Input: part model. Units: mm. Frame: model coordinates. A direction names the side the tool comes from. Round coordinates to 2 decimals unless told otherwise and drop trailing zeros. Order: outer loops, then holes, each group sorted by start corner. A loop starts at its lowest first (then second) coordinate and runs counter-clockwise, first axis right, second up. Notation, with made-up numbers: (54.5, 10.5) -> (64.5, 10.5) arc R21 cw to (64.5, 19.5) -> close; hole circle Ø2 at (-32.75, 42). An arc over 180 degrees is marked (long way). Answer as CSV lines item,"result". Start each with the question number.
1) Mould query, pull axis X, two halves, no side actions, for faces 4 (the face through (0, 5, 35)), 5 (the face through (5, 5, 65)), 6 (the face through (5, 0, 35)). Classes: +X half, -X half, draft (parallel to the pull), parting line (faces both ways), or undercut.
2) Section query D-D, the plane x = 5. Output: boundary loops of the cut face in (y, z), and give its area (3 significant figures).
3) Access query for faces 1 (the face through (6.6, 6.2, 68)), 2 (the face through (7, 5, 3)), 3 (the face through (7.2, 5.1, 0)). Directions: +Z, -Z, +X, -X, +Y, -Y. A direction counts if a zero-diameter tool reaches every point of the face in a straight line with its end or side. Return the directions, or none.
4) First-contact query: P1, Ø1.2, axis at x = 5.5, y = 5.5, coming from the -Z side; P2, Ø1, axis at x = 6, z = 54.5, coming from the -Y side; P3, Ø2.5, axis at y = 5.7, z = 55.6, coming from the +X side; P4, Ø1.5, axis at x = 6, y = 5.5, coming from the +Z side. Flat tips, straight axial feed; report the tip coordinate or a pass-through.
5) Section query A-A, the plane z = 55.6. Output: boundary loops of the cut face in (x, y).
6) Line query: L1, parallel to Y at x = 3.75, z = 12; L2, parallel to X at y = 5, z = 66.85; L3, parallel to Z at x = 4, y = 7. Output: solid intervals per line, ascending.
7) Section query C-C, the plane y = 5. Output: boundary loops of the cut face in (x, z).
8) Section query B-B, the plane x = 1.75. Output: boundary loops of the cut face in (y, z), and give its area (3 significant figures).
```python
from build123d import *

# Parameters (mm, degrees)
ESQUISSE1_W             = 10
ESQUISSE1_H             = 10
BOSS_EXTRU_1_DEPTH      = 71
ESQUISSE2_R             = 2
ENL_V_MAT_EXTRU_1_DEPTH = 73.394751191
ESQUISSE3_R             = 2
ENL_V_MAT_EXTRU_2_DEPTH = 6
ENL_V_START             = -6
ESQUISSE4_R             = 2
ENL_V_MAT_EXTRU_3_DEPTH = 6


with BuildPart() as part:
    # Esquisse1 → Boss.-Extru.1 (new body)
    with BuildSketch(Plane.XY):
        with Locations((5, 5)):
            Rectangle(ESQUISSE1_W, ESQUISSE1_H)
    extrude(amount=BOSS_EXTRU_1_DEPTH)

    # Esquisse2 → Enlèv. mat.-Extru.1 (cut, through all)
    with BuildSketch(Plane.ZY):
        with Locations((12, 5.7)):
            Circle(ESQUISSE2_R)
        with Locations((55.6, 5.7)):
            Circle(ESQUISSE2_R)
    extrude(amount=-ENL_V_MAT_EXTRU_1_DEPTH, mode=Mode.SUBTRACT)

    # Esquisse3 → Enlèv. mat.-Extru.2 (cut)
    with BuildSketch(Plane(origin=(0, 0, 0), x_dir=(-1, 0, 0), z_dir=(0, 0, -1))):
        with Locations((-5, 5)):
            Circle(ESQUISSE3_R)
    extrude(amount=-ENL_V_MAT_EXTRU_2_DEPTH, mode=Mode.SUBTRACT)

    # Esquisse4 → Enlèv. mat.-Extru.3 (cut)
    with BuildSketch(Plane.XY.offset(71).offset(ENL_V_START)):
        with Locations(Location((5, 5, 0), (0, 0, 180))):
            Circle(ESQUISSE4_R)
    extrude(amount=ENL_V_MAT_EXTRU_3_DEPTH, mode=Mode.SUBTRACT)


solid = part.part
```
Findings:
1,face 4,"-X half"
1,face 5,"undercut"
1,face 6,"draft"
2,outline,"(0, 0) -> (3, 0) -> (3, 6) -> (7, 6) -> (7, 0) -> (10, 0) -> (10, 71) -> (7, 71) -> (7, 65) -> (3, 65) -> (3, 71) -> (0, 71) -> close; hole circle Ø4 at (5.7, 12); hole circle Ø4 at (5.7, 55.6)"
2,area,"637 mm^2"
3,face 1,"+Z"
3,face 2,"-Z"
3,face 3,"-Z, +X, -X, +Y, -Y"
4,P1,"stops at z = 6"
4,P2,"stops at y = 0"
4,P3,"passes through"
4,P4,"stops at z = 65"
5,outline,"(0, 0) -> (10, 0) -> (10, 3.7) -> (0, 3.7) -> close; (0, 7.7) -> (10, 7.7) -> (10, 10) -> (0, 10) -> close"
6,L1,"y = 0 to 3.7, 7.7 to 10"
6,L2,"x = 0 to 3, 7 to 10"
6,L3,"z = 0 to 10.48, 13.52 to 54.08, 57.12 to 71"
7,outline,"(0, 0) -> (3, 0) -> (3, 6) -> (7, 6) -> (7, 0) -> (10, 0) -> (10, 10.13) -> (0, 10.13) -> close; (0, 13.87) -> (10, 13.87) -> (10, 53.73) -> (0, 53.73) -> close; (0, 57.47) -> (10, 57.47) -> (10, 71) -> (7, 71) -> (7, 65) -> (3, 65) -> (3, 71) -> (0, 71) -> close"
8,outline,"(0, 0) -> (10, 0) -> (10, 71) -> (0, 71) -> close; hole circle Ø4 at (5.7, 12); hole circle Ø4 at (5.7, 55.6)"
8,area,"685 mm^2"
